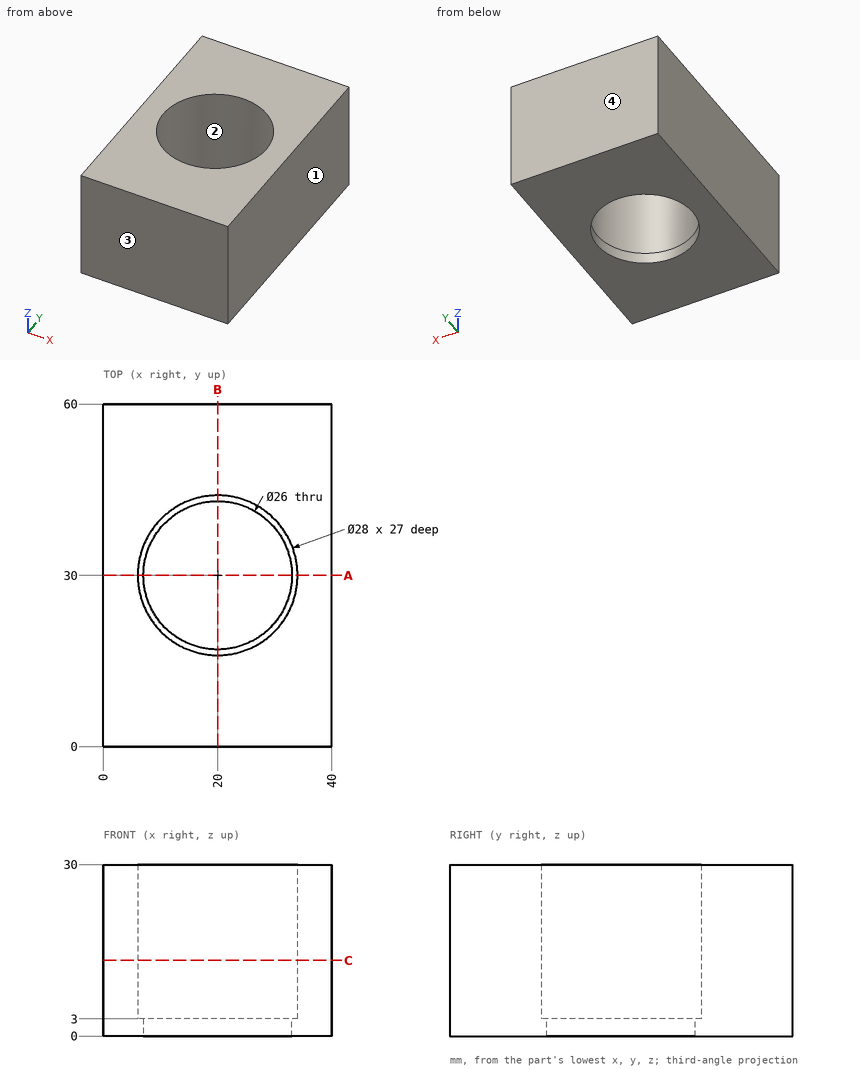
Geometry check sheet. Reference: drawing and pictorial views, mm from the part's lowest x, y, z. Coordinates: 2 decimals unless noted, no trailing zeros. Order: outer loops, then holes, each group sorted by start corner. A loop starts at its lowest first (then second) coordinate and runs counter-clockwise, first axis right, second up. Notation, with made-up numbers: M 80,-33 L 122,-33 A29 ccw 122,3 Z; hole C -4.5,52 d8. An arc over 180 degrees is marked long. Return JSON: item names as keys, results as strings.
1) Release check for a two-part mould opening along Y. For the marked faces 1, 2, 3 and 4 record: +Y half, -Y half, draft (parallel to the pull), parting line (faces both ways), or undercut.
Answer list:
{"face 1": "draft", "face 2": "undercut", "face 3": "-Y half", "face 4": "+Y half"}
2) Cross-section at B-B, the plane x = 20. Record the boundary of the cut face in (y, z), and give its area (3 significant figures).
Answer list:
{"outline": "M 0,0 L 17,0 L 17,3 L 16,3 L 16,30 L 0,30 Z; M 43,0 L 60,0 L 60,30 L 44,30 L 44,3 L 43,3 Z", "area": "966 mm2"}
3) Cross-section at C-C, the plane z = 13.25. Record the boundary of the cut face in (x, y), and give its area (3 significant figures).
Answer list:
{"outline": "M 0,0 L 40,0 L 40,60 L 0,60 Z; hole C 20,30 d28", "area": "1,780 mm2"}
4) Thickness scan on L1, parallel to Y at x = 20, z = 1.8; L2, parallel to Y at x = 20, z = 14.75; L3, parallel to Z at x = 10, y = 21. Record the ranges inside material, lowest first. Write a range as [from, to].
Answer list:
{"L1": "[0, 17], [43, 60]", "L2": "[0, 16], [44, 60]", "L3": "[0, 3]"}
5) Cross-section at A-A, the plane y = 30. Record the boundary of the cut face in (x, z), and give its area (3 significant figures).
Answer list:
{"outline": "M 0,0 L 7,0 L 7,3 L 6,3 L 6,30 L 0,30 Z; M 33,0 L 40,0 L 40,30 L 34,30 L 34,3 L 33,3 Z", "area": "366 mm2"}
6) Gauge pin test, flat end, axial feed: pin 1 (3 mm diameter, centred on x = 29, y = 12, fed in from -Z). Record the tip position at first contact, or that the pin passes through.
Answer list:
{"pin 1": "z = 0"}
